Here's how the part is built. I have some questions about the finished solid (model axes, mm). Face numbers are marked on the shaded views. A direction names the side the tool comes from. Coordinates: 2 decimals unless noted, no trailing zeros. Write each loop counter-clockwise with the first axis right and the second up, starting at its lowest first coordinate (ties: lowest second). Pieces come first, ordered by that corner, then holes.
Item 1: For the marked faces 1, 2 and 3, which set-ups out of +Z, -Z, +X, -X, +Y, -Y let a thin tool reach every point of the face, with its end or its side?
Item 2: I want a section at D-D (y = 16). Please give me the cut outline in (x, z).
Item 3: I'm going to push flat-ended pins straight in: P1, Ø3, axis at x = -12, z = 1.5, coming from the +Y side; P2, Ø3, axis at x = 2.5, y = -1.5, coming from the -Z side; P3, Ø1.9, axis at x = 0, y = 0, coming from the +Z side; P4, Ø12, axis at x = -17, z = 1, coming from the +Y side. Where does each tip first touch, or does it pass through?
Item 4: I want a section at C-C (z = 8.25). Please give me the cut outline in (x, y), and give its area (3 significant figures).
Item 5: If we mould it in two halves opening along X, with no side actions, what happens to the marked faces 4, 5 and 6? For each: pulls with the +X half, pulls with the -X half, needs draft (parallel to the pull), parting line crosses it, or undercut.
Item 6: I want a section at A-A (y = 0). Please give me the cut outline in (x, z) (3 decimals), and give its area (3 significant figures).
Item 7: Please list where these lines run through material, in increasing order: line 1 (Y direction, x = 0, z = -3.75) (3 decimals); line 2 (Y direction, x = 0, z = 6.5); line 3 (Z direction, x = -18, y = -4).
from build123d import *

# Parameters (mm, degrees)
SKETCH1_R           = 25
BOSS_EXTRUDE1_DEPTH = 1.5
SKETCH2_R           = 25
SKETCH2_R_2         = 20
BOSS_EXTRUDE2_DEPTH = 10
SKETCH3_R           = 5
BOSS_EXTRUDE3_DEPTH = 5
SKETCH4_R           = 1.585
CUT_EXTRUDE1_DEPTH  = 10


with BuildPart() as part:
    # Sketch1 → Boss-Extrude1 (new, symmetric)
    with BuildSketch(Plane.XY):
        Circle(SKETCH1_R)
    extrude(amount=BOSS_EXTRUDE1_DEPTH, both=True)

    # Sketch2 → Boss-Extrude2 (add, symmetric)
    with BuildSketch(Plane.XY):
        Circle(SKETCH2_R)
        Circle(SKETCH2_R_2, mode=Mode.SUBTRACT)
    extrude(amount=BOSS_EXTRUDE2_DEPTH, both=True)

    # Sketch3 → Boss-Extrude3 (add, symmetric)
    with BuildSketch(Plane.XY):
        Circle(SKETCH3_R)
    extrude(amount=BOSS_EXTRUDE3_DEPTH, both=True)

    # Sketch4 → Cut-Extrude1 (cut)
    with BuildSketch(Plane(origin=(0, 0, -5), x_dir=(-1, 0, 0), z_dir=(0, 0, -1))):
        Circle(SKETCH4_R)
    extrude(amount=-CUT_EXTRUDE1_DEPTH, mode=Mode.SUBTRACT)


solid = part.part
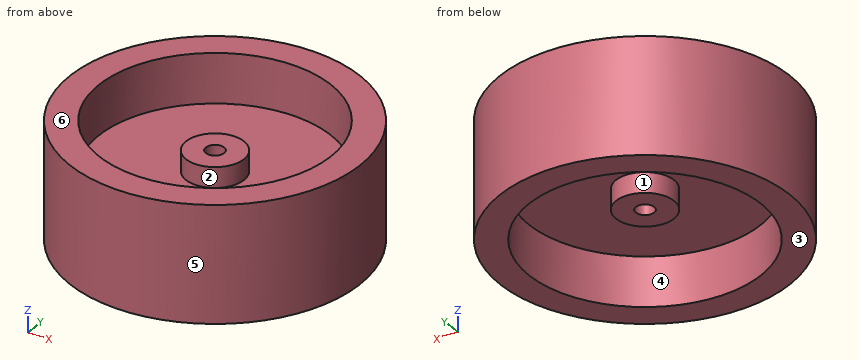
Answer:
1. face 1: -Z
1. face 2: +Z
1. face 3: -Z, +X, -X, +Y, -Y
2. outline: (-19.21, -10) - (-12, -10) - (-12, -1.5) - (12, -1.5) - (12, -10) - (19.21, -10) - (19.21, 10) - (12, 10) - (12, 1.5) - (-12, 1.5) - (-12, 10) - (-19.21, 10) - close
3. P1: stops at y = 22.69
3. P2: stops at z = -5
3. P3: passes through
3. P4: stops at y = 22.45
4. outline: circle Ø50 at (0, 0); hole circle Ø40 at (0, 0)
4. area: 707 mm2
5. face 4: undercut
5. face 5: parting line crosses it
5. face 6: needs draft
6. outline: (-25, -10) - (-20, -10) - (-20, -1.5) - (-5, -1.5) - (-5, -5) - (-1.585, -5) - (-1.585, 5) - (-5, 5) - (-5, 1.5) - (-20, 1.5) - (-20, 10) - (-25, 10) - close; (1.585, -5) - (5, -5) - (5, -1.5) - (20, -1.5) - (20, -10) - (25, -10) - (25, 10) - (20, 10) - (20, 1.5) - (5, 1.5) - (5, 5) - (1.585, 5) - close
6. area: 358 mm2
7. line 1: y = -25 to -20, -5 to -1.585, 1.585 to 5, 20 to 25
7. line 2: y = -25 to -20, 20 to 25
7. line 3: z = -1.5 to 1.5
